Source: CAD feature listing. Evaluate the final solid. Frame: model axes, mm. Coordinates: 2 decimals unless noted, no trailing zeros. Write each loop counter-clockwise with the first axis right and the second up, starting at its lowest first coordinate (ties: lowest second). Pieces come first, ordered by that corner, then holes. Notation, with made-up numbers: (89.5, -23) - (119.5, -23) arc R12 cw to (119.5, -3) - close; hole circle Ø10 at (-19.5, 44.25). An arc over 180 degrees is marked (long way). One line per item, written item: value.
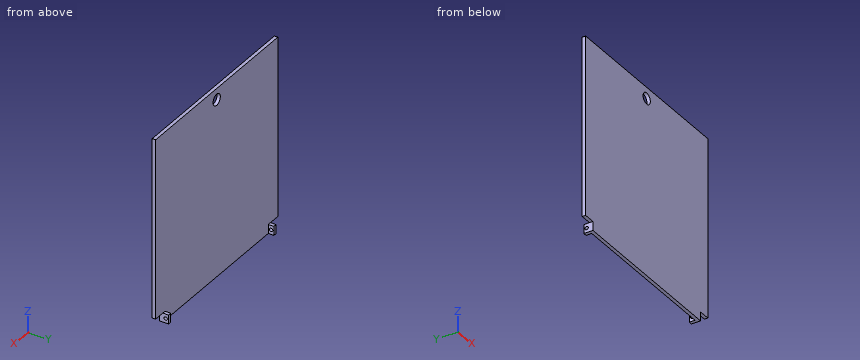
Autodesk Inventor part; units mm, degrees
ref_plane "YZ Plane" through (0, 0, 0) normal (1, 0, 0) x (0, 1, 0)
ref_plane "XZ Plane" through (0, 0, 0) normal (0, 1, 0) x (-1, 0, 0)
ref_plane "XY Plane" through (0, 0, 0) normal (0, 0, 1) x (1, 0, 0)
sketch "Náčrt1" plane through (0, 0, 0) normal (0, 1, 0) x (-1, 0, 0)
  line L0 (84, 84) -> (-84, 84)
  line L1 (-84, 84) -> (-84, -84)
  line L2 (-84, -84) -> (84, -84)
  line L3 (84, -84) -> (84, 84)
  line L4 (0, -117.6) -> (0, 117.6)
  line L5 (-117.6, 0) -> (117.6, 0)
  point P0 (0, 0)
  dimension "d0" = 168
  dimension "d1" = 168
extrude "Vysunutí1" add sketch "Náčrt1" along normal mid plane 3
sketch "Náčrt2" plane through (0, 1.5, 0) normal (0, 1, 0) x (1, 0, 0)
  line L0 (-84, -84) -> (84, -84)
  line L1 (84, -84) -> (84, 84)
  point P0 (0, 0)
  point P1 (0, -74)
  dimension "d13" = 10
  dimension "d14" = 84
sketch "Náčrt3" plane through (0, 1.5, 0) normal (0, 1, 0) x (1, 0, 0)
  line L0 (74, 84) -> (84, 84)
  line L1 (84, 84) -> (84, 76)
  line L2 (84, 76) -> (74, 76)
  line L3 (74, 76) -> (74, 84)
  line L4 (84, 84) -> (-84, 84)
  line L5 (84, -84) -> (84, 84)
  point P0 (0, 0)
  dimension "d9" = 10
  dimension "d10" = 8
extrude "Vysunutí3" cut sketch "Náčrt3" against normal through all
mirror "Zrcadlit1" about plane through (0, 0, 0) normal (1, 0, 0) of "Vysunutí3"
hole "Díra1" at (0, 1.5, 74) direction (0, -1, 0) diameter 10 end through all
sketch "Náčrt4" plane through (0, 1.5, 0) normal (0, 1, 0) x (1, 0, 0)
  line L0 (71, 76) -> (74, 76)
  line L1 (74, 76) -> (74, 84)
  line L2 (74, 84) -> (71, 84)
  line L3 (71, 84) -> (71, 76)
  line L4 (74, 76) -> (74, 84)
  line L5 (74, 84) -> (-74, 84)
  point P0 (0, 0)
  dimension "d22" = 3
extrude "Vysunutí4" add sketch "Náčrt4" along normal blind 5
sketch "Náčrt5" plane through (74, -1.5, -76) normal (1, 0, 0) x (0, 0, -1)
  line L0 (0, 8) -> (8, 8)
  line L1 (0, 3) -> (0, 8)
  line L2 (8, 8) -> (8, 0)
  point P0 (-76, 1.5)
  point P1 (4, 5.5)
  dimension "d25" = 2.5
  dimension "d34" = 4
hole "Díra2" at (74, 4, -80) direction (-1, 0, 0) diameter 3 depth 3
mirror "Zrcadlit2" about plane through (0, 0, 0) normal (1, 0, 0) of "Vysunutí4", "Díra2"
properties part number "Cabinet - door"
1) Material intervals for line 1 (Y direction, x = -71.55, z = -80); line 2 (X direction, y = -0.5, z = 74); line 3 (Z direction, x = 0, y = 0.05), sorted ascending.
Values found:
line 1: -1.5 to 2.5, 5.5 to 6.5
line 2: -84 to -5, 5 to 84
line 3: -84 to 69, 79 to 84
2) Section query C-C on x = 0. Output: boundary loops of the cut face in (y, z).
Values found:
outline: (-1.5, -84) - (1.5, -84) - (1.5, 69) - (-1.5, 69) - close; (-1.5, 79) - (1.5, 79) - (1.5, 84) - (-1.5, 84) - close
3) Section query B-B on z = 74. Output: boundary loops of the cut face in (x, y), then the cut area to 3 significant figures.
Values found:
outline: (-84, -1.5) - (-5, -1.5) - (-5, 1.5) - (-84, 1.5) - close; (5, -1.5) - (84, -1.5) - (84, 1.5) - (5, 1.5) - close
area: 474 mm2
4) Contact query for flat-ended pins moving along their axis: P1, Ø4, axis at y = 3, z = -79.5, coming from the +X side; P2, Ø3.5, axis at x = -72, y = 4, coming from the +Z side; P3, Ø4, axis at y = 4, z = -80, coming from the -X side; P4, Ø3.5, axis at x = 72, y = 3, coming from the +Z side. Output: stop coordinate, or through.
Values found:
P1: x = 74
P2: z = -76
P3: x = -74
P4: z = 84
5) Section query A-A on y = 4. Output: boundary loops of the cut face in (x, z).
Values found:
outline: (-74, -84) - (-71, -84) - (-71, -81.5) - (-74, -81.5) - close; (-74, -78.5) - (-71, -78.5) - (-71, -76) - (-74, -76) - close; (71, -84) - (74, -84) - (74, -81.5) - (71, -81.5) - close; (71, -78.5) - (74, -78.5) - (74, -76) - (71, -76) - close
6) Section query D-D on x = -56. Output: boundary loops of the cut face in (y, z), then the cut area to 3 significant figures.
Values found:
outline: (-1.5, -84) - (1.5, -84) - (1.5, 84) - (-1.5, 84) - close
area: 504 mm2
